The model under review builds one solid part; all positions refer to its coordinate system, in mm. Face numbers are marked on the shaded views. A direction names the side the tool comes from. Round coordinates to 2 decimals unless told otherwise and drop trailing zeros. Loops run counter-clockwise (first coordinate to the right, second up) from the corner with the lowest first, then second, coordinate; pieces in that order, holes last. Notation, with made-up numbers: (10, -12) - (42, -12) arc R4 ccw to (42, -6) - close; hole circle Ø5 at (72, 46.25). An arc over 180 degrees is marked (long way). Answer as CSV lines item,"result".
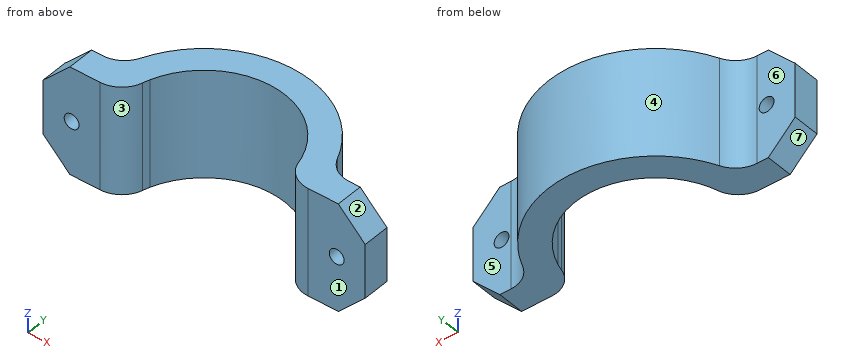
from build123d import *

# Parameters (mm, degrees)
F1_DEPTH  = 50.8
F3_DEPTH  = 12.7
F4_SIZE   = 12.7
F5_R      = 11.35
F5_R_2    = 10
F6_DEPTH  = 44.45
F7_R      = 12.7
F8_R      = 3.5
F9_DEPTH  = 50.801
F10_W     = 183.8439181447
F10_H     = 157.3934331536
F11_DEPTH = 114.3
F12_R     = 12.7


with BuildPart() as f1:
    # F0 (on Top) → F1 (new body)
    with BuildSketch(Plane.XY):
        with BuildLine():
            ThreePointArc((-35.9210244843, 12.7), (0, 38.1), (35.9210244843, 12.7))
            Line((35.9210244843, 12.7), (49.1868884968, 12.7))
            ThreePointArc((49.1868884968, 12.7), (0, 50.8), (-49.1868884968, 12.7))
            Line((-49.1868884968, 12.7), (-35.9210244843, 12.7))
        make_face()
        with BuildLine():
            ThreePointArc((-49.1868884968, -12.7), (-50.8, 0), (-49.1868884968, 12.7))
            Line((-49.1868884968, 12.7), (-76.2, 12.7))
            Line((-76.2, 12.7), (-76.2, -12.7))
            Line((-76.2, -12.7), (-49.1868884968, -12.7))
        make_face()
        with BuildLine():
            ThreePointArc((-35.9210244843, -12.7), (-38.1, 0), (-35.9210244843, 12.7))
            Line((-35.9210244843, 12.7), (-49.1868884968, 12.7))
            ThreePointArc((-49.1868884968, 12.7), (-50.8, 0), (-49.1868884968, -12.7))
            Line((-49.1868884968, -12.7), (-35.9210244843, -12.7))
        make_face()
        with BuildLine():
            ThreePointArc((35.9210244843, 12.7), (37.5513051228, 6.4427853895), (38.1, 0))
            ThreePointArc((38.1, 0), (37.5513051228, -6.4427853895), (35.9210244843, -12.7))
            Line((35.9210244843, -12.7), (49.1868884968, -12.7))
            ThreePointArc((49.1868884968, -12.7), (50.3951085704, -6.4010180581), (50.8, 0))
            ThreePointArc((50.8, 0), (50.3951085704, 6.4010180581), (49.1868884968, 12.7))
            Line((49.1868884968, 12.7), (35.9210244843, 12.7))
        make_face()
        with BuildLine():
            Line((76.2, 12.7), (49.1868884968, 12.7))
            ThreePointArc((49.1868884968, 12.7), (50.3951085704, 6.4010180581), (50.8, 0))
            ThreePointArc((50.8, 0), (50.3951085704, -6.4010180581), (49.1868884968, -12.7))
            Line((49.1868884968, -12.7), (76.2, -12.7))
            Line((76.2, -12.7), (76.2, 12.7))
        make_face()
        with BuildLine():
            ThreePointArc((-19.05, -32.9955678842), (-29.2989914869, -24.3552683798), (-35.9210244843, -12.7))
            Line((-35.9210244843, -12.7), (-49.1868884968, -12.7))
            ThreePointArc((-49.1868884968, -12.7), (-38.2071387235, -33.479165918), (-19.05, -47.0928603931))
            Line((-19.05, -47.0928603931), (-19.05, -32.9955678842))
        make_face()
        with BuildLine():
            Line((49.1868884968, -12.7), (35.9210244843, -12.7))
            ThreePointArc((35.9210244843, -12.7), (29.2989914869, -24.3552683798), (19.05, -32.9955678842))
            Line((19.05, -32.9955678842), (19.05, -47.0928603931))
            ThreePointArc((19.05, -47.0928603931), (38.2071387235, -33.479165918), (49.1868884968, -12.7))
        make_face()
        with BuildLine():
            Line((19.05, -47.0928603931), (19.05, -32.9955678842))
            ThreePointArc((19.05, -32.9955678842), (0, -38.1), (-19.05, -32.9955678842))
            Line((-19.05, -32.9955678842), (-19.05, -47.0928603931))
            ThreePointArc((-19.05, -47.0928603931), (0, -50.8), (19.05, -47.0928603931))
        make_face()
        with BuildLine():
            Line((19.05, -88.9), (19.05, -47.0928603931))
            ThreePointArc((19.05, -47.0928603931), (0, -50.8), (-19.05, -47.0928603931))
            Line((-19.05, -47.0928603931), (-19.05, -88.9))
            Line((-19.05, -88.9), (19.05, -88.9))
        make_face()
    extrude(amount=F1_DEPTH)

    # F2 (on face) → F3 (cut)
    with BuildSketch(Plane.XZ.offset(12.7)):
        Polygon((-55.6935602012, 25.3597094836), (-59.1586096141, 31.4419321502), (-66.1584936613, 31.4822226666), (-69.6933282956, 25.4402905164), (-66.2282788827, 19.3580678498), (-59.2283948355, 19.3177773334), align=None)
        Polygon((59.1938884968, 31.4621778265), (55.6938884968, 25.4), (59.1938884968, 19.3378221735), (66.1938884968, 19.3378221735), (69.6938884968, 25.4), (66.1938884968, 31.4621778265), align=None)
    extrude(amount=-F3_DEPTH, mode=Mode.SUBTRACT)

    # F4
    f4_edges = [f1.edges().sort_by_distance(p)[0] for p in [
        (-76.2, 0, 50.8),
        (-76.2, 0, 0),
        (76.2, 0, 50.8),
        (76.2, 0, 0),
    ]]
    chamfer(f4_edges, length=F4_SIZE)

    # F5 (on face) → F6 (cut)
    with BuildSketch(Plane.XY.offset(50.8)):
        with Locations((0, -67.9964301965)):
            Circle(F5_R)
        with Locations((0, -67.9964301965)):
            Circle(F5_R_2, mode=Mode.SUBTRACT)
    extrude(amount=-F6_DEPTH, mode=Mode.SUBTRACT)

    # F7
    f7_edges = [f1.edges().sort_by_distance(p)[0] for p in [
        (-19.05, -88.9, 25.4),
        (19.05, -88.9, 25.4),
        (-19.05, -47.09286, 25.4),
        (19.05, -47.09286, 25.4),
        (49.186888, -12.7, 25.4),
        (-49.186888, -12.7, 25.4),
        (-49.186888, 12.7, 25.4),
        (49.186888, 12.7, 25.4),
    ]]
    fillet(f7_edges, radius=F7_R)

    # F8 (on face) → F9 (cut, through all)
    with BuildSketch(Plane.XZ):
        with Locations((-62.6585516377, 25.4402905164)):
            Circle(F8_R)
        with Locations((62.6938884968, 25.4402905164)):
            Circle(F8_R)
    extrude(amount=-F9_DEPTH, mode=Mode.SUBTRACT)

    # F10 (on Front) → F11 (cut)
    with BuildSketch(Plane.XZ):
        with Locations((-6.0164444149, -2.5229565799)):
            Rectangle(F10_W, F10_H)
    extrude(amount=F11_DEPTH, mode=Mode.SUBTRACT)

    # F12
    f12_edges = [f1.edges().sort_by_distance(p)[0] for p in [
        (-38.1, 0, 25.4),
        (38.1, 0, 25.4),
    ]]
    fillet(f12_edges, radius=F12_R)


solid = f1.part
1. Take a section at D-D (z = 46.5). State the section outline as (x, y) points (3 decimals), plus the area to 3 significant figures.
Numbers:
outline,"(-67.8, 0) - (-49.187, 0) arc R12.7 ccw to (-36.89, 9.525) arc R38.1 cw to (36.89, 9.525) arc R12.7 ccw to (49.187, 0) - (67.8, 0) - (67.8, 12.7) - (58.199, 12.7) arc R12.7 cw to (46.559, 20.32) arc R50.8 ccw to (-46.559, 20.32) arc R12.7 cw to (-58.199, 12.7) - (-67.8, 12.7) - close"
area,"2,200 mm²"
2. Draft analysis for pull direction X (two halves, no side actions). For the marked faces 1, 2, 3 and 4, state which applies: +X half, -X half, draft (parallel to the pull), parting line (faces both ways), or undercut.
Numbers:
face 1,"draft"
face 2,"+X half"
face 3,"undercut"
face 4,"parting line"
3. Take a section at A-A (z = 36). State the section outline as (x, y) points (3 decimals), plus the area to 3 significant figures.
Numbers:
outline,"(-76.2, 0) - (-49.187, 0) arc R12.7 ccw to (-36.89, 9.525) arc R38.1 cw to (36.89, 9.525) arc R12.7 ccw to (49.187, 0) - (76.2, 0) - (76.2, 12.7) - (58.199, 12.7) arc R12.7 cw to (46.559, 20.32) arc R50.8 ccw to (-46.559, 20.32) arc R12.7 cw to (-58.199, 12.7) - (-76.2, 12.7) - close"
area,"2,410 mm²"
4. Take a section at B-B (y = 22). State the section outline as (x, z) points, plus the area to 3 significant figures.
Numbers:
outline,"(-45.79, 0) - (-31.11, 0) - (-31.11, 50.8) - (-45.79, 50.8) - close; (31.11, 0) - (45.79, 0) - (45.79, 50.8) - (31.11, 50.8) - close"
area,"1,490 mm²"
5. Clearance check with flat-ended pins moving along their axes: pin 1 (12 mm diameter, centred on x = 2, y = 35.5, fed in from +Z); pin 2 (2 mm diameter, centred on y = 40.5, z = 40, fed in from -X); pin 3 (11 mm diameter, centred on x = 62.69, z = 25.44, fed in from +Y); pin 4 (1.5 mm diameter, centred on x = -29.5, z = 23.5, fed in from +Y). State where each tip first meets the part, or that it passes through.
Numbers:
pin 1,"stops at z = 50.8"
pin 2,"stops at x = -31.94"
pin 3,"stops at y = 12.74"
pin 4,"stops at y = 41.88"
6. Take a section at C-C (x = 61). State the section outline as (y, z) points, plus the area to 3 significant figures.
Numbers:
outline,"(0, 0) - (12.7, 0) - (12.7, 22.38) - (0, 22.38) - close; (0, 28.5) - (12.7, 28.5) - (12.7, 50.8) - (0, 50.8) - close"
area,"567 mm²"
7. Wall thickness on probe 1 along Y at (x, z) = (-65, 3); probe 2 along X at (y, z) = (27.5, 33); probe 3 along X at (y, z) = (11, 48.5): over which ranges is each line inside the solid? List them lowest first.
Numbers:
probe 1,"y = 0 to 12.7"
probe 2,"x = -42.71 to -26.37, 26.37 to 42.71"
probe 3,"x = -65.8 to -36.48, 36.48 to 65.8"
8. Tool access review of the marked faces 5, 6 and 7: name each direction out of +Z, -Z, +X, -X, +Y, -Y from which nothing blocks a thin tool from reaching the whole face with its end or side.
Numbers:
face 5,"+Z, -Z, +X, +Y"
face 6,"+Z, -Z, -X, +Y"
face 7,"-Z, -X, +Y, -Y"
